Part print with two shaded views. Sizes in mm from the minimum x, y, z corner. A direction names the side the tool comes from. Give positions to 0.01 mm unless a question says otherwise; leave off trailing zeros. Write each loop counter-clockwise with the first axis right and the second up, starting at its lowest first coordinate (ties: lowest second). Pieces come first, ordered by that corner, then holes.
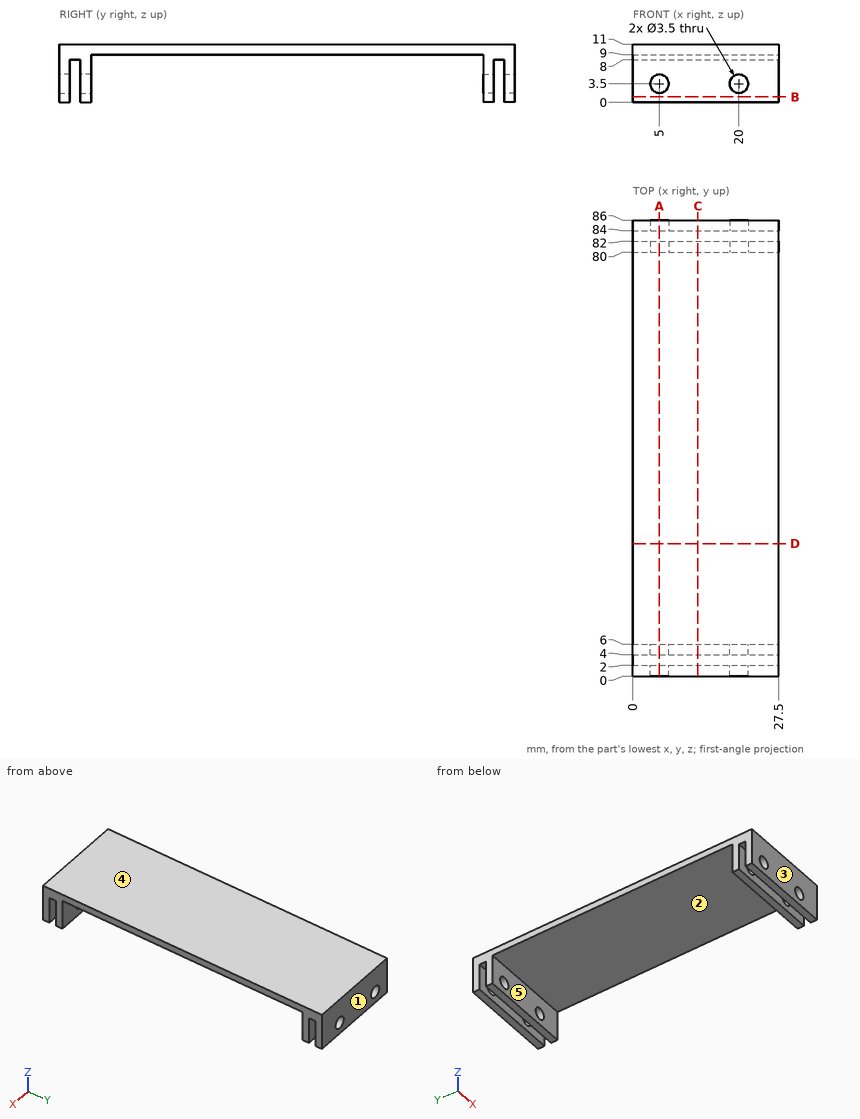
1) Pin check, flat tips, straight feed: pin 1 Ø10 at (x, y) = (19, 23.5) entering from -Z; pin 2 Ø5 at (x, z) = (12.5, 8) entering from -Y; pin 3 Ø3 at (x, z) = (5, 3.5) entering from -Y. Stop position of each tip, or through.
Answers follow:
pin 1: stops at z = 9
pin 2: stops at y = 0
pin 3: passes through
2) Saw through at C-C, the plane x = 12.25. Write the cut outline in (y, z).
Answers follow:
outline: (0, 0) - (2, 0) - (2, 8) - (4, 8) - (4, 0) - (6, 0) - (6, 9) - (80, 9) - (80, 0) - (82, 0) - (82, 8) - (84, 8) - (84, 0) - (86, 0) - (86, 11) - (0, 11) - close
3) Saw through at A-A, the plane x = 5. Count the separate pieces of the cut face and the enclosed holes in it, then the cut area to 3 significant figures.
Answers follow:
separate pieces: 5
enclosed holes: 0
area: 220 mm2
4) Saw through at D-D, the plane y = 25. Write the cut outline in (x, z).
Answers follow:
outline: (0, 9) - (27.5, 9) - (27.5, 11) - (0, 11) - close
5) Wall check: L1, parallel to Y at x = 13.75, z = 7.5; L2, parallel to X at y = 1.5, z = 3.5; L3, parallel to Z at x = 20, y = 85.6. Give the ranges that are in metal, low to high.
Answers follow:
L1: y = 0 to 2, 4 to 6, 80 to 82, 84 to 86
L2: x = 0 to 3.25, 6.75 to 18.25, 21.75 to 27.5
L3: z = 0 to 1.75, 5.25 to 11
6) Two-plate mould, pull along Y, no slides. Class the marked faces 3, 4 and 5: +Y half, -Y half, draft (parallel to the pull), parting line (faces both ways), or undercut.
Answers follow:
face 3: -Y half
face 4: draft
face 5: undercut
7) 3-axis set-ups, long thin cutter, end or side, ignore diameter. For the marked faces 1 and 2: which of +Z, -Z, +X, -X, +Y, -Y reach the whole face in a straight line?
Answers follow:
face 1: +Z, -Z, +X, -X, +Y
face 2: -Z, +X, -X
8) Saw through at B-B, the plane z = 1. Write the cut outline in (x, y).
Answers follow:
outline: (0, 0) - (27.5, 0) - (27.5, 2) - (0, 2) - close; (0, 4) - (27.5, 4) - (27.5, 6) - (0, 6) - close; (0, 80) - (27.5, 80) - (27.5, 82) - (0, 82) - close; (0, 84) - (27.5, 84) - (27.5, 86) - (0, 86) - close
